```python
from build123d import *

# Parameters (mm, degrees)
F0_W     = 65.532
F0_H     = 136.652
F1_DEPTH = 7.62
F2_T     = -1.27
F3_R     = 2.54


with BuildPart() as f1:
    # F0 (on Front) → F1 (new body)
    with BuildSketch(Plane.XZ):
        Rectangle(F0_W, F0_H)
    extrude(amount=F1_DEPTH)

    # F2
    f2_openings = [f1.faces().sort_by_distance(p)[0] for p in [
        (0, -7.62, 0),
    ]]
    offset(amount=F2_T, openings=f2_openings)

    # F3
    f3_edges = [f1.edges().sort_by_distance(p)[0] for p in [
        (-32.766, -3.81, -68.326),
        (32.766, -3.81, -68.326),
        (32.766, -3.81, 68.326),
        (-32.766, -3.81, 68.326),
    ]]
    fillet(f3_edges, radius=F3_R)


solid = f1.part
```
Design review of the part built by this model. Coordinates are the model's own, in mm. A direction names the side the tool comes from. Round coordinates to 2 decimals unless told otherwise and drop trailing zeros. Write each loop counter-clockwise with the first axis right and the second up, starting at its lowest first coordinate (ties: lowest second). Pieces come first, ordered by that corner, then holes. Notation, with made-up numbers: (6.5, 41.25) -> (28.5, 41.25) arc R22 cw to (28.5, 48.25) -> close; hole circle Ø3 at (-29.75, 29.5). An arc over 180 degrees is marked (long way). Answer in a Markdown table with one row per item.
Q1. For faces 4 (the face through (32.002, -3.863, -67.602)), 5 (the face through (0, -4, -67.056)), list the 3-axis set-ups (+Z, -Z, +X, -X, +Y, -Y) from which the entire face can be reached by the end or side of a thin tool; tool diameter is ignored.
The answers:
| item | result |
|---|---|
| face 4 | -Z, +X, +Y, -Y |
| face 5 | -Y |
Q2. Clearance check with a flat-ended pin moving along its axis: pin 1 Ø1 at (x, z) = (-15.5, -17) entering from -Y. State where the tip first meets the part, or that it passes through.
The answers:
| item | result |
|---|---|
| pin 1 | y = -1.27 |
Q3. Take a section at C-C, the plane x = 15. State the section outline as (y, z) points.
The answers:
| item | result |
|---|---|
| outline | (-7.62, -68.33) -> (0, -68.33) -> (0, 68.33) -> (-7.62, 68.33) -> (-7.62, 67.06) -> (-1.27, 67.06) -> (-1.27, -67.06) -> (-7.62, -67.06) -> close |
Q4. Take a section at B-B, the plane z = -34. State the section outline as (x, y) points.
The answers:
| item | result |
|---|---|
| outline | (-32.77, -7.62) -> (-31.5, -7.62) -> (-31.5, -1.27) -> (31.5, -1.27) -> (31.5, -7.62) -> (32.77, -7.62) -> (32.77, 0) -> (-32.77, 0) -> close |
Q5. Take a section at A-A, the plane y = -5.75. State the section outline as (x, z) points, then the cut area to 3 significant figures.
The answers:
| item | result |
|---|---|
| outline | (-32.77, -65.79) arc R2.54 ccw to (-30.23, -68.33) -> (30.23, -68.33) arc R2.54 ccw to (32.77, -65.79) -> (32.77, 65.79) arc R2.54 ccw to (30.23, 68.33) -> (-30.23, 68.33) arc R2.54 ccw to (-32.77, 65.79) -> close; hole (-31.5, -67.06) -> (31.5, -67.06) -> (31.5, 67.06) -> (-31.5, 67.06) -> close |
| area | 502 mm² |
Q6. Draft analysis for pull direction X (two halves, no side actions). For faces 1 (the face through (0, -4, 67.056)), 2 (the face through (-32.766, -4, -1)), 3 (the face through (32.042, -3.863, 67.562)), state which applies: +X half, -X half, draft (parallel to the pull), parting line (faces both ways), or undercut.
The answers:
| item | result |
|---|---|
| face 1 | undercut |
| face 2 | -X half |
| face 3 | +X half |
Q7. To check wall thickness, follow L1, parallel to X at y = -2, z = -9.5; L2, parallel to Z at x = 14, y = -4.25; L3, parallel to Y at x = 15.5, z = 61. State the ranges of each line that lie inside material, in increasing order. Write a range as [from, to].
The answers:
| item | result |
|---|---|
| L1 | [-32.77, -31.5], [31.5, 32.77] |
| L2 | [-68.33, -67.06], [67.06, 68.33] |
| L3 | [-1.27, 0] |
